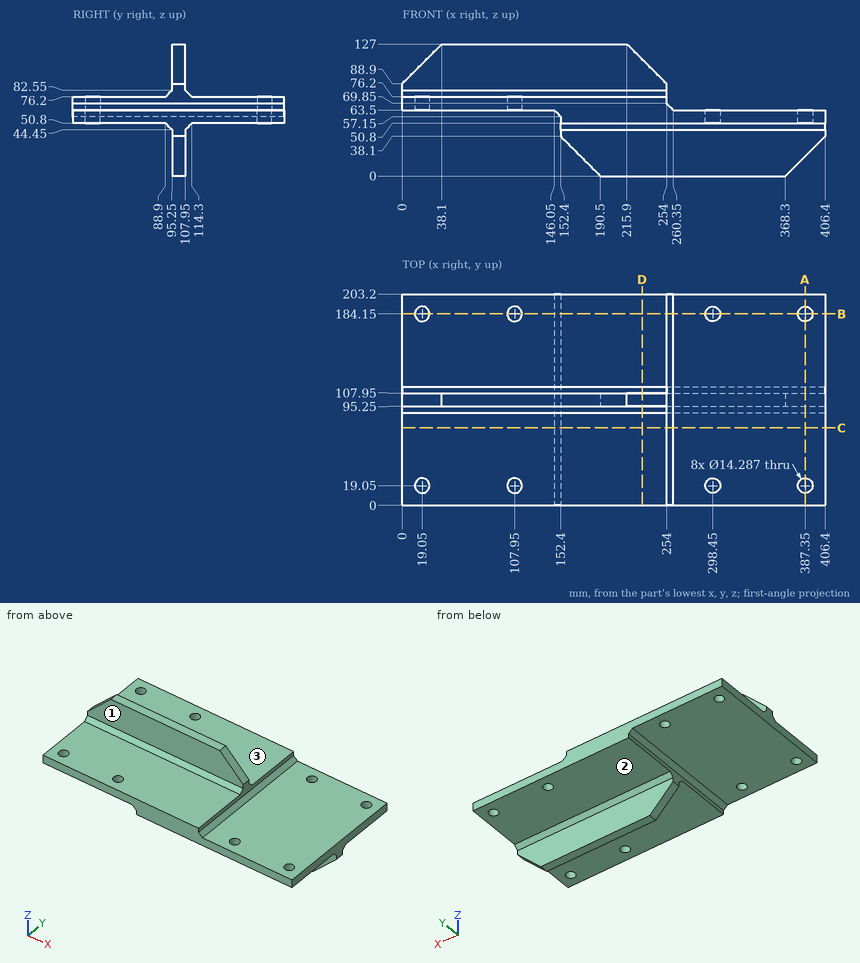
The figure shows three views and two pictorial views of one solid part (mm, origin at its lowest corner). Answer the questions. A direction names the side the tool comes from. Give positions to 0.01 mm unless a question says otherwise; leave off trailing zeros. Write each loop counter-clockwise with the first axis right and the second up, starting at its lowest first coordinate (ties: lowest second). Pieces come first, ordered by that corner, then holes. Notation, with made-up numbers: M -9.75,46.5 L 49.25,46.5 A7 ccw 49.25,53.5 Z; hole C 2,-14.5 d7. An arc over 180 degrees is marked long. One line per item, written item: value. Start each with the question number.
(1) Find section C-C (y = 74.5). Determine the outline of the cut face in (x, z), plus the area to 3 significant figures.
(2) Flat-ended cylindrical pins translate along their axes: pin 1 Ø9.5 at (y, z) = (116.5, 78) entering from +X; pin 2 Ø1.5 at (x, y) = (252, 156) entering from -Z; pin 3 Ø12 at (x, y) = (92.5, 118) entering from -Z; pin 4 Ø11.5 at (x, y) = (298.45, 19.05) entering from +Z. Find the tip coordinate at first contact, or state that the pin passes through.
(3) Find section D-D (x = 230.5). Determine the outline of the cut face in (y, z), plus the area to 3 significant figures.
(4) Find section A-A (x = 387.35). Determine the outline of the cut face in (y, z).
(5) Find section B-B (y = 184.15). Determine the outline of the cut face in (x, z), plus the area to 3 significant figures.
(6) Find the intervals of material crossed by line 1 (X direction, y = 19, z = 70); line 2 (Y direction, x = 107.95, z = 67.75); line 3 (Z direction, x = 60, y = 11.5), in increasing order.
(7) A tool of negligible diameter and unlimited length cuts with its end or side. For the marked faces 1, 2 and 3, from which of +Z, -Z, +X, -X, +Y, -Y can it reach the whole face along a straight path? Write none if from no direction.
Results below:
1. outline: M 0,63.5 L 146.05,63.5 L 152.4,57.15 L 152.4,50.8 L 406.4,50.8 L 406.4,63.5 L 260.35,63.5 L 254,69.85 L 254,76.2 L 0,76.2 Z
1. area: 6,490 mm^2
2. pin 1: stops at x = 254
2. pin 2: stops at z = 50.8
2. pin 3: stops at z = 63.5
2. pin 4: passes through
3. outline: M 0,50.8 L 88.9,50.8 L 95.25,44.45 L 95.25,0 L 107.95,0 L 107.95,44.45 L 114.3,50.8 L 203.2,50.8 L 203.2,76.2 L 114.3,76.2 L 107.95,82.55 L 107.95,112.4 L 95.25,112.4 L 95.25,82.55 L 88.9,76.2 L 0,76.2 Z
3. area: 6,350 mm^2
4. outline: M 0,50.8 L 11.91,50.8 L 11.91,63.5 L 0,63.5 Z; M 26.19,50.8 L 88.9,50.8 L 95.25,44.45 L 95.25,19.05 L 107.95,19.05 L 107.95,44.45 L 114.3,50.8 L 177.01,50.8 L 177.01,63.5 L 26.19,63.5 Z; M 191.29,50.8 L 203.2,50.8 L 203.2,63.5 L 191.29,63.5 Z
5. outline: M 0,63.5 L 11.91,63.5 L 11.91,76.2 L 0,76.2 Z; M 26.19,63.5 L 100.81,63.5 L 100.81,76.2 L 26.19,76.2 Z; M 115.09,63.5 L 146.05,63.5 L 152.4,57.15 L 152.4,50.8 L 291.31,50.8 L 291.31,63.5 L 260.35,63.5 L 254,69.85 L 254,76.2 L 115.09,76.2 Z; M 305.59,50.8 L 380.21,50.8 L 380.21,63.5 L 305.59,63.5 Z; M 394.49,50.8 L 406.4,50.8 L 406.4,63.5 L 394.49,63.5 Z
5. area: 5,770 mm^2
6. line 1: x = 0 to 11.91, 26.19 to 100.81, 115.09 to 254
6. line 2: y = 0 to 11.91, 26.19 to 177.01, 191.29 to 203.2
6. line 3: z = 63.5 to 76.2
7. face 1: +Z, +X, -X, -Y
7. face 2: -Z, +X, -X, +Y
7. face 3: +Z, +X, -X, +Y
